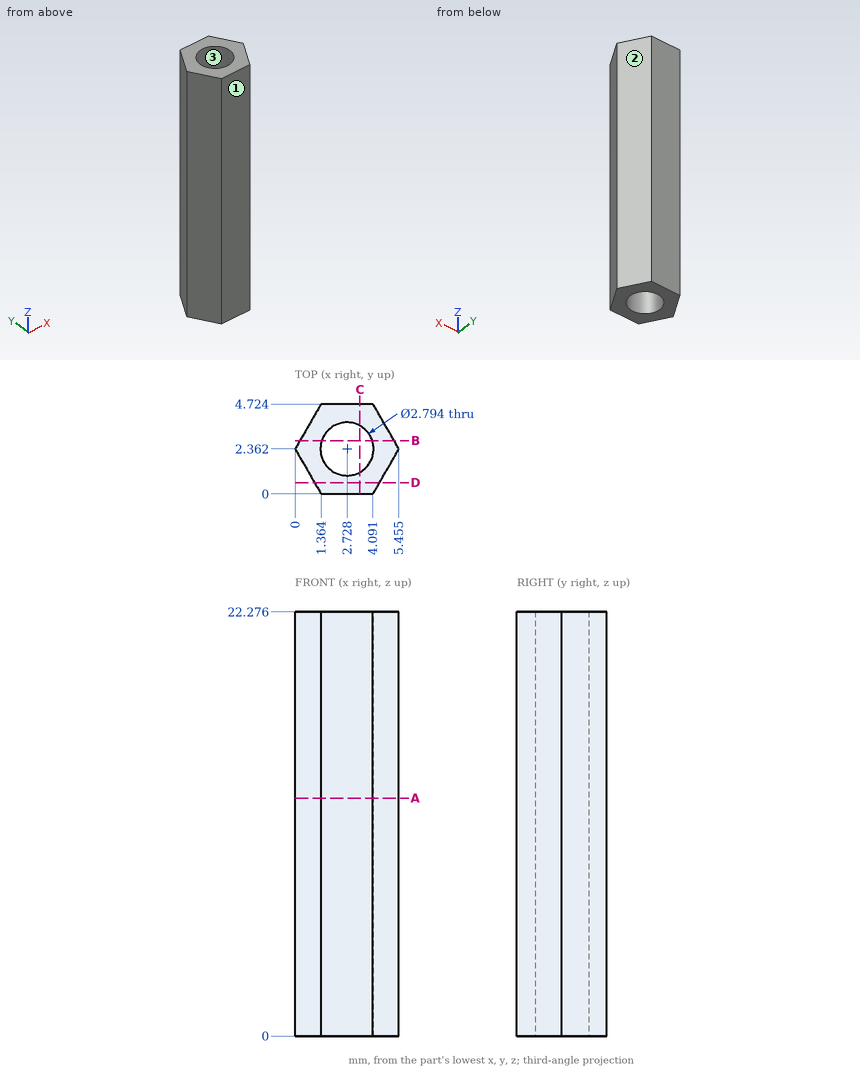
Source: three-view drawing plus pictorial views. Frame: mm from the lowest corner of the part. Coordinates: 2 decimals unless noted, no trailing zeros. Loops run counter-clockwise (first coordinate to the right, second up) from the corner with the lowest first, then second, coordinate; pieces in that order, holes last. Notation, with made-up numbers: (46.25, 9.25) - (65.25, 9.25) arc R17 ccw to (65.25, 35.25) - close; hole circle Ø4 at (-28, 21.5). An arc over 180 degrees is marked (long way). One line per question, with ' | ' between items.
1) Pull-direction query (Y, two-part tool) for the marked faces 1, 2 and 3; classes: released by +Y, released by -Y, zero draft, split by the parting line, or undercut.
Report:
face 1: released by -Y | face 2: released by +Y | face 3: undercut
2) Section D-D, the plane y = 0.6. Return loops of the section in (x, z) (1 decimal).
Report:
outline: (1, 0) - (4.4, 0) - (4.4, 22.3) - (1, 22.3) - close
3) Section C-C, the plane x = 3.4. Return loops of the section in (y, z) (1 decimal).
Report:
outline: (0, 0) - (1.1, 0) - (1.1, 22.3) - (0, 22.3) - close; (3.6, 0) - (4.7, 0) - (4.7, 22.3) - (3.6, 22.3) - close
4) Section B-B, the plane y = 2.8. Return loops of the section in (x, z) (1 decimal).
Report:
outline: (0.3, 0) - (1.4, 0) - (1.4, 22.3) - (0.3, 22.3) - close; (4.1, 0) - (5.2, 0) - (5.2, 22.3) - (4.1, 22.3) - close
5) First-contact query: P1, Ø1, axis at x = 3, y = 2, coming from the -Z side; P2, Ø1.5, axis at y = 1.5, z = 16, coming from the +X side. Flat tips, straight axial feed; report the tip coordinate or a pass-through.
Report:
P1: passes through | P2: stops at x = 5.39
6) Section A-A, the plane z = 12.5. Return loops of the section in (x, y) (1 decimal), then the cut area to 3 significant figures.
Report:
outline: (0, 2.4) - (1.4, 0) - (4.1, 0) - (5.5, 2.4) - (4.1, 4.7) - (1.4, 4.7) - close; hole circle Ø2.8 at (2.7, 2.4) | area: 13.2 mm²
7) Line query: line 1 along X through (y, z) = (1.75, 9) (1 decimal); line 2 along Y through (x, z) = (1.95, 19.5) (1 decimal); line 3 along Y through (x, z) = (3.95, 20.5) (1 decimal). Output: solid intervals per line, ascending.
Report:
line 1: x = 0.4 to 1.5, 4 to 5.1 | line 2: y = 0 to 1.2, 3.5 to 4.7 | line 3: y = 0 to 1.7, 3 to 4.7
